from build123d import *

# Parameters (mm, degrees)
ESQUISSE1_W             = 98
ESQUISSE1_H             = 173
ESQUISSE1_W_2           = 20
ESQUISSE1_H_2           = 8
BOSS_EXTRU_1_DEPTH      = 6
ESQUISSE2_W             = 10
ESQUISSE2_H             = 6
BOSS_EXTRU_2_DEPTH      = 6
ESQUISSE3_R             = 1.5
ENL_V_MAT_EXTRU_1_DEPTH = 6
ESQUISSE4_W             = 20
ESQUISSE4_H             = 6
ESQUISSE4_W_2           = 28
ESQUISSE4_H_2           = 10
ENL_V_MAT_EXTRU_2_DEPTH = 6


with BuildPart() as part:
    # Esquisse1 → Boss.-Extru.1 (new body)
    with BuildSketch(Plane.XY):
        Rectangle(ESQUISSE1_W, ESQUISSE1_H)
        with Locations((30, -22.5)):
            Rectangle(ESQUISSE1_W_2, ESQUISSE1_H_2, mode=Mode.SUBTRACT)
        with Locations((-30, -22.5)):
            Rectangle(ESQUISSE1_W_2, ESQUISSE1_H_2, mode=Mode.SUBTRACT)
    extrude(amount=BOSS_EXTRU_1_DEPTH)

    # Esquisse2 → Boss.-Extru.2 (add)
    with BuildSketch(Plane.XY.offset(6)):
        with Locations((24.5, -89.5)):
            Rectangle(ESQUISSE2_W, ESQUISSE2_H)
        with Locations((-24.5, -89.5)):
            Rectangle(ESQUISSE2_W, ESQUISSE2_H)
    extrude(amount=-BOSS_EXTRU_2_DEPTH)

    # Esquisse3 → Enlèv. mat.-Extru.1 (cut)
    with BuildSketch(Plane.XY.offset(6)):
        with Locations((-15, 83.5)):
            Circle(ESQUISSE3_R)
        with Locations((24.5, -89.5)):
            Circle(ESQUISSE3_R)
        with Locations((-24.5, -89.5)):
            Circle(ESQUISSE3_R)
        with Locations((15, 83.5)):
            Circle(ESQUISSE3_R)
    extrude(amount=-ENL_V_MAT_EXTRU_1_DEPTH, mode=Mode.SUBTRACT)

    # Esquisse4 → Enlèv. mat.-Extru.2 (cut)
    with BuildSketch(Plane.XY.offset(6)):
        with Locations((0, 83.5)):
            Rectangle(ESQUISSE4_W, ESQUISSE4_H)
        with Locations((0, -81.5)):
            Rectangle(ESQUISSE4_W_2, ESQUISSE4_H_2)
    extrude(amount=-ENL_V_MAT_EXTRU_2_DEPTH, mode=Mode.SUBTRACT)


solid = part.part
Source: CAD feature listing. Evaluate the final solid. Frame: model axes, mm. A direction names the side the tool comes from. Round coordinates to 2 decimals unless told otherwise and drop trailing zeros. Write each loop counter-clockwise with the first axis right and the second up, starting at its lowest first coordinate (ties: lowest second). Pieces come first, ordered by that corner, then holes. Notation, with made-up numbers: M 68.25,64.25 L 88.25,64.25 A21 ccw 88.25,98.25 Z; hole C -36.75,81 d3. An arc over 180 degrees is marked long. One line per item, written item: value. Start each with the question number.
Item 1: Section query A-A (x = 38). Return the cut outline in (y, z).
Item 2: Section query B-B (y = -78.5). Return the cut outline in (x, z).
Item 3: Section query C-C (z = 2.75). State how many separate pieces and enclosed holes the cut face has, plus the area to 3 significant figures.
Item 4: Pin query (flat end, axial travel): pin 1 (3 mm diameter, centred on x = -17, z = 3, fed in from -Y); pin 2 (4 mm diameter, centred on x = -24, y = 0, fed in from -Z). Return the tip coordinate at first contact, or that it passes through.
Item 5: Mould query, pull axis X, two halves, no side actions, for faces 1 (the flat face through (-49, -1, 3)), 2 (the flat face through (39, -86.5, 3)), 3 (the flat face through (19.5, -90, 3)), 4 (the flat face through (-30, -18.5, 3)). Classes: pulls with the +X half, pulls with the -X half, needs draft (parallel to the pull), parting line crosses it, or undercut.
Item 6: Set-up query: faces 5 (the flat face through (-19.5, -90, 3)), 6 (the flat face through (-39, -86.5, 3)), 7 (the flat face through (-10, 83, 3)). Return all of +Z, -Z, +X, -X, +Y, -Y with unobstructed straight access to the full face (end or side cutting, diameter ignored); none if empty.
Item 7: Ray query, L1, parallel to Y at x = 24.5, z = 2.8; L2, parallel to Y at x = -35, z = 1.65; L3, parallel to X at y = -89.5, z = 1.35. Return the intervals inside material, ascending. Write a range as from..to.
Result set:
1. outline: M -86.5,0 L -26.5,0 L -26.5,6 L -86.5,6 Z; M -18.5,0 L 86.5,0 L 86.5,6 L -18.5,6 Z
2. outline: M -49,0 L -14,0 L -14,6 L -49,6 Z; M 14,0 L 49,0 L 49,6 L 14,6 Z
3. separate pieces: 1
3. enclosed holes: 6
3. area: 16,300 mm²
4. pin 1: stops at y = -86.5
4. pin 2: stops at z = 0
5. face 1: pulls with the -X half
5. face 2: needs draft
5. face 3: undercut
5. face 4: undercut
6. face 5: +Z, -Z, -Y
6. face 6: +Z, -Z, -X, -Y
6. face 7: +Z, -Z, +Y
7. L1: y = -92.5..-91, -88..-26.5, -18.5..86.5
7. L2: y = -86.5..-26.5, -18.5..86.5
7. L3: x = -29.5..-26, -23..-19.5, 19.5..23, 26..29.5
